from build123d import *

# Parameters (mm, degrees)
SKETCH1_R           = 20.193
BOSS_EXTRUDE1_DEPTH = 28.194
SKETCH2_R           = 20.193
SKETCH3_R           = 14.478
SKETCH4_R           = 3.175
BOSS_EXTRUDE2_DEPTH = 27.94
SKETCH5_R           = 26.3525
BOSS_EXTRUDE4_DEPTH = 9.4488
SKETCH6_OUTSIDE_W   = 76.102
SKETCH6_OUTSIDE_H   = 76.102
SKETCH6_OUTSIDE_R   = 25.3365
CUT_EXTRUDE1_DEPTH  = 5.08
SKETCH9_R           = 29.21
SKETCH10_R          = 29.21
BOSS_EXTRUDE5_DEPTH = 15.24
SKETCH11_R          = 31.496
BOSS_EXTRUDE6_DEPTH = 2.54
SKETCH14_R          = 22.225
SKETCH12_R          = 20.32
SKETCH15_W          = 18.542
SKETCH15_H          = 6.35
BOSS_EXTRUDE7_DEPTH = 43.18
SKETCH16_W          = 18.542
SKETCH16_H          = 2.032
CUT_EXTRUDE2_DEPTH  = 15.748
SKETCH17_R          = 5.461
BOSS_EXTRUDE8_DEPTH = 10.16
BOSS_EXTRUDE8_TAPER = 1
CUT_EXTRUDE3_REACH  = 89.162
FILLET1_R           = 10.16
FILLET3_R           = 10.16
SKETCH20_W          = 4.6355
SKETCH20_H          = 7.2136
BOSS_EXTRUDE9_DEPTH = 31.75


with BuildPart() as part:
    # Sketch1 → Boss-Extrude1 (new body)
    with BuildSketch(Plane(origin=(0, 0, 0), x_dir=(0, 0, -1), z_dir=(1, 0, 0))):
        Circle(SKETCH1_R)
    extrude(amount=BOSS_EXTRUDE1_DEPTH)

    # Sketch2 → Loft2 section 0
    with BuildSketch(Plane(origin=(28.194, 0, 0), x_dir=(0, 0, -1), z_dir=(1, 0, 0))):
        Circle(SKETCH2_R)
    # Sketch3 → Loft2 section 1
    with BuildSketch(Plane(origin=(39.37, 0, 0), x_dir=(0, 0, -1), z_dir=(1, 0, 0))):
        Circle(SKETCH3_R)
    loft()

    # Sketch4 → Boss-Extrude2 (add)
    with BuildSketch(Plane(origin=(39.37, 0, 0), x_dir=(0, 0, -1), z_dir=(1, 0, 0))):
        Circle(SKETCH4_R)
    extrude(amount=BOSS_EXTRUDE2_DEPTH)

    # Sketch5 → Boss-Extrude4 (add)
    with BuildSketch(Plane(origin=(0, 0, 0), x_dir=(0, 0, -1), z_dir=(1, 0, 0))):
        Circle(SKETCH5_R)
    extrude(amount=-BOSS_EXTRUDE4_DEPTH)

    # Sketch6 outside → Cut-Extrude1 (cut)
    with BuildSketch(Plane.ZY.offset(9.4488)):
        Rectangle(SKETCH6_OUTSIDE_W, SKETCH6_OUTSIDE_H)
        Circle(SKETCH6_OUTSIDE_R, mode=Mode.SUBTRACT)
    extrude(amount=-CUT_EXTRUDE1_DEPTH, mode=Mode.SUBTRACT)

    # Sketch9 → section 0 of loft3
    with BuildSketch(Plane.ZY.offset(11.9888), mode=Mode.PRIVATE) as loft3_s0:
        Circle(SKETCH9_R)
    # loft up to a face of the part (loft3)
    loft([loft3_s0.sketch, Face(Wire([part.edges().sort_by_distance((-9.4488, 18.469513629, -17.344027749))[0]]))])

    # Sketch10 → Boss-Extrude5 (add)
    with BuildSketch(Plane.ZY.offset(11.9888)):
        with Locations(Location((0, 0, 0), (0, 0, 180))):
            Circle(SKETCH10_R)
    extrude(amount=BOSS_EXTRUDE5_DEPTH)

    # Sketch11 → Boss-Extrude6 (add)
    with BuildSketch(Plane.ZY.offset(27.2288)):
        Circle(SKETCH11_R)
    extrude(amount=BOSS_EXTRUDE6_DEPTH)

    # Sketch14 → Loft6 section 0
    with BuildSketch(Plane.ZY.offset(29.7688)):
        Circle(SKETCH14_R)
    # Sketch12 → Loft6 section 1
    with BuildSketch(Plane.ZY.offset(37.3888)):
        Circle(SKETCH12_R)
    loft()

    # Sketch15 → Boss-Extrude7 (add, symmetric)
    with BuildSketch(Plane.XY):
        with Locations((-39.0398, 0)):
            Rectangle(SKETCH15_W, SKETCH15_H)
    extrude(amount=BOSS_EXTRUDE7_DEPTH, both=True)

    # Sketch16 → Cut-Extrude2 (cut)
    with BuildSketch(Plane.XY.offset(43.18)):
        with Locations((-39.0398, 2.159)):
            Rectangle(SKETCH16_W, SKETCH16_H)
        with Locations((-39.0398, -2.159)):
            Rectangle(SKETCH16_W, SKETCH16_H)
    cut_extrude2 = extrude(amount=-CUT_EXTRUDE2_DEPTH, mode=Mode.SUBTRACT)

    # Mirror1: Cut-Extrude2 across plane
    add(cut_extrude2.mirror(Plane.XY), mode=Mode.SUBTRACT)

    # Sketch17 → Boss-Extrude8 (add)
    with BuildSketch(Plane.ZY.offset(37.3888)):
        with Locations((0, -11.811)):
            Circle(SKETCH17_R)
    extrude(amount=BOSS_EXTRUDE8_DEPTH, taper=BOSS_EXTRUDE8_TAPER)

    # Sketch18 → Cut-Extrude3 (cut, up to next)
    with BuildSketch(Plane(origin=(0, 3.175, 0), x_dir=(1, 0, 0), z_dir=(0, 1, 0)), mode=Mode.PRIVATE) as cut_extrude3_sk1:
        with BuildLine():
            Line((-48.3108, 23.940709333), (-48.3108, -23.940709333))
            ThreePointArc((-48.3108, -23.940709333), (-43.18, 0), (-48.3108, 23.940709333))
        make_face()
    cut_extrude3_tool1 = extrude(cut_extrude3_sk1.sketch, amount=-CUT_EXTRUDE3_REACH, mode=Mode.PRIVATE) & part.part
    add(cut_extrude3_tool1.solids().sort_by_distance((-46.250554, 3.175, 0))[0], mode=Mode.SUBTRACT)

    # Fillet1
    fillet1_edges = [part.edges().sort_by_distance(p)[0] for p in [
        (-48.3108, 0, -43.18),
    ]]
    fillet(fillet1_edges, radius=FILLET1_R)

    # Fillet3
    fillet3_edges = [part.edges().sort_by_distance(p)[0] for p in [
        (-48.3108, 0, 43.18),
    ]]
    fillet(fillet3_edges, radius=FILLET3_R)

    # Sketch20 → Boss-Extrude9 (add, symmetric)
    with BuildSketch(Plane(origin=(0, 0, 0), x_dir=(-1, 0, 0), z_dir=(0, -0.25881904510250753, -0.9659258262890719))):
        with Locations((15.51305, 0)):
            Rectangle(SKETCH20_W, SKETCH20_H)
    extrude(amount=BOSS_EXTRUDE9_DEPTH, both=True)


solid = part.part
Work out the finished part from the listing and answer in its coordinate system (mm). A direction names the side the tool comes from. Round coordinates to 2 decimals unless told otherwise and drop trailing zeros. Write each loop counter-clockwise with the first axis right and the second up, starting at its lowest first coordinate (ties: lowest second). Pieces come first, ordered by that corner, then holes. Notation, with made-up numbers: (36, 46.25) -> (44, 46.25) arc R20 ccw to (44, 50.25) -> close; hole circle Ø3 at (-32.5, 8). An arc over 180 degrees is marked (long way). Write each question's results on one line, items separated by ' | '.
Item 1: Which of the six approach directions +Z, -Z, +X, -X, +Y, -Y give full straight-line access (tool end or side, diameter ignored) to faces 1 (the face through (0, -15, -14)), 2 (the face through (-6.944, 21.364, 13.621)), 3 (the face through (-37.389, -6, 0)), 4 (the face through (-39, -1.143, 35)), 5 (the face through (-39, 1.143, -35))?
Result set:
face 1: +X | face 2: none | face 3: -X | face 4: +Z, -X, -Y | face 5: -Z, -X, +Y
Item 2: A cutting plane is placed at C-C, the plane x = 11. Determine the outline of the cut face in (y, z).
Result set:
outline: circle Ø40.39 at (0, 0)
Item 3: Find the intervals of material crossed by line 1 along X through (y, z) = (8, 2); line 2 along X through (y, z) = (4, -29.5); line 3 along Y through (x, z) = (-11, 0), in increasing order. Write a range as [from, to].
Result set:
line 1: [-37.39, 39.37] | line 2: [-29.77, -27.23] | line 3: [-27.7, 27.7]
Item 4: The mould has two halves that part along Z. Classify faces 6 (the face through (-15.48, 11.34, 28.38)), 7 (the face through (-48.311, 0, 28)), 8 (the face through (13.9, -19.713, 4.377)): +Z half, -Z half, draft (parallel to the pull), parting line (faces both ways), or undercut.
Result set:
face 6: undercut | face 7: draft | face 8: parting line
Item 5: A cutting plane is placed at A-A, the plane x = -35. Determine the outline of the cut face in (y, z) (3 decimals).
Result set:
outline: (-3.175, -27.432) -> (-1.143, -27.432) -> (-1.143, -43.18) -> (1.143, -43.18) -> (1.143, -27.432) -> (3.175, -27.432) -> (3.175, -20.675) arc R20.917 ccw to (3.175, 20.675) -> (3.175, 27.432) -> (1.143, 27.432) -> (1.143, 43.18) -> (-1.143, 43.18) -> (-1.143, 27.432) -> (-3.175, 27.432) -> (-3.175, 20.675) arc R20.917 ccw to (-3.175, -20.675) -> close
Item 6: A cutting plane is placed at B-B, the plane z = 36. Determine the outline of the cut face in (x, y).
Result set:
outline: (-47.86, -1.14) -> (-29.77, -1.14) -> (-29.77, 1.14) -> (-47.86, 1.14) -> close
Item 7: Flat-ended cylindrical pins translate along their axes: P1, Ø8, axis at x = -42.5, z = 35, coming from the -Y side; P2, Ø2.5, axis at y = -7, z = -29.5, coming from the -X side; P3, Ø1.1, axis at y = 0, z = -35.5, coming from the +X side; P4, Ø5, axis at x = 42, z = -7, coming from the +Y side. Find the tip coordinate at first contact, or state that the pin passes through.
Result set:
P1: y = -1.14 | P2: x = -29.77 | P3: x = -29.77 | P4: through
